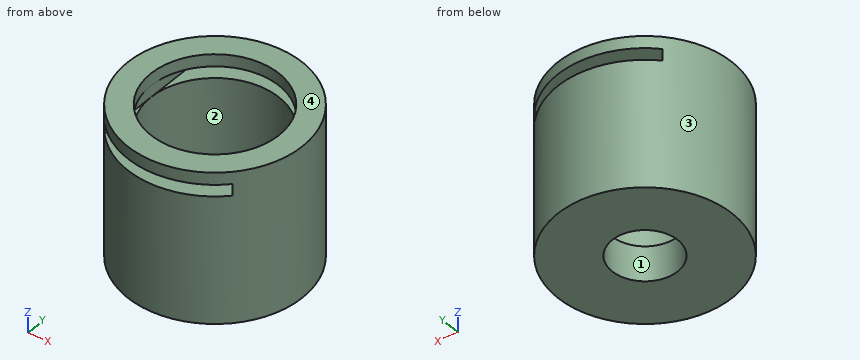
```python
from build123d import *

# Parameters (mm, degrees)
SKETCH1_R               = 15
BOSS_EXTRUDE5_DEPTH     = 26
SKETCH3_R               = 5.625
CUT_EXTRUDE2_DEPTH      = 34.555923471
SKETCH4_R               = 11
CUT_EXTRUDE3_DEPTH      = 20
CUT_EXTRUDE4_DEPTH      = 34.555923471
CUT_EXTRUDE4_DEPTH_BACK = 34.555923471
SKETCH6_W               = 22
SKETCH6_H               = 2
CUT_EXTRUDE6_START      = 6
SKETCH7_R               = 11
SKETCH7_R_2             = 9
CUT_EXTRUDE6_DEPTH      = 2


with BuildPart() as part:
    # Sketch1 → Boss-Extrude5 (new body)
    with BuildSketch(Plane.XY):
        Circle(SKETCH1_R)
    extrude(amount=BOSS_EXTRUDE5_DEPTH)

    # Sketch3 → Cut-Extrude2 (cut, through all)
    with BuildSketch(Plane.XY.offset(26)):
        Circle(SKETCH3_R)
    extrude(amount=-CUT_EXTRUDE2_DEPTH, mode=Mode.SUBTRACT)

    # Sketch4 → Cut-Extrude3 (cut)
    with BuildSketch(Plane.XY.offset(26)):
        Circle(SKETCH4_R)
    extrude(amount=-CUT_EXTRUDE3_DEPTH, mode=Mode.SUBTRACT)

    # Sketch6 → Cut-Extrude4 (cut, two sides: drawn at the far end of the back side and taken through both)
    with BuildSketch(Plane(origin=(0, 0, 0), x_dir=(1, 0, 0), z_dir=(0, 1, 0)).offset(-CUT_EXTRUDE4_DEPTH_BACK)):
        with Locations((0, -22.90958557)):
            Rectangle(SKETCH6_W, SKETCH6_H)
    extrude(amount=CUT_EXTRUDE4_DEPTH + CUT_EXTRUDE4_DEPTH_BACK, mode=Mode.SUBTRACT)

    # Sketch7 → Cut-Extrude6 (cut)
    with BuildSketch(Plane.XY.offset(CUT_EXTRUDE6_START)):
        Circle(SKETCH7_R)
        Circle(SKETCH7_R_2, mode=Mode.SUBTRACT)
    extrude(amount=-CUT_EXTRUDE6_DEPTH, mode=Mode.SUBTRACT)


solid = part.part
```
CAD build for the part. Positions are in the model's coordinates, mm. Face numbers are marked on the shaded views. Round coordinates to 2 decimals unless told otherwise and drop trailing zeros. Loops run counter-clockwise (first coordinate to the right, second up) from the corner with the lowest first, then second, coordinate; pieces in that order, holes last. Notation, with made-up numbers: M -17.5,-33 L 39.5,-33 A32 cw 39.5,4 Z; hole C 81.25,26 d9. An arc over 180 degrees is marked long. Use a Markdown table: item, result. Add a question column.
(1) Cut at C-C (z = 23.5). Give the cut face in (x, y), and give its area (3 significant figures).
(2) Cut at D-D (x = 9.5). Give the cut face in (y, z), and give its area (3 significant figures).
(3) Pull direction X, two halves, no side cores. Call the marked faces 1, 2, 3 and 4: +X half, -X half, draft (parallel to the pull), parting line (faces both ways), or undercut.
(4) Drill centre lines: line 1 (Y direction, x = 0, z = 4.6) (3 decimals); line 2 (Y direction, x = 0, z = 17.5); line 3 (Z direction, x = -6.25, y = -13.5). Where is each one in solid material? Low to high.
(5) Flat gauge pins, fed straight in: pin 1 (12 mm diameter, centred on x = 10, z = 10.5, fed in from +Y); pin 2 (12 mm diameter, centred on x = -2, y = -10, fed in from +Z); pin 3 (2 mm diameter, centred on y = 4.5, z = 23, fed in from +X); pin 4 (2 mm diameter, centred on y = 2, z = 15, fed in from +X). Where does each tip first touch, or does it go through?
(6) Cut at A-A (x = 0). Give the cut face in (y, z) (3 decimals).
Geometry says:
| question | item | result |
|---|---|---|
| 1 | outline | M -11,-10.2 L -11,10.2 A15 ccw Z; M 11,-10.2 A15 ccw 11,10.2 Z |
| 1 | area | 112 mm² |
| 2 | outline | M -11.61,0 L 11.61,0 L 11.61,21.91 L 5.55,21.91 L 5.55,4 L -5.55,4 L -5.55,21.91 L -11.61,21.91 Z; M -11.61,23.91 L -5.55,23.91 L -5.55,26 L -11.61,26 Z; M 5.55,23.91 L 11.61,23.91 L 11.61,26 L 5.55,26 Z |
| 2 | area | 335 mm² |
| 3 | face 1 | undercut |
| 3 | face 2 | undercut |
| 3 | face 3 | parting line |
| 3 | face 4 | draft |
| 4 | line 1 | y = -15 to -11, -9 to -5.625, 5.625 to 9, 11 to 15 |
| 4 | line 2 | y = -15 to -11, 11 to 15 |
| 4 | line 3 | z = 0 to 21.91, 23.91 to 26 |
| 5 | pin 1 | stops at y = 14.46 |
| 5 | pin 2 | stops at z = 26 |
| 5 | pin 3 | stops at x = 14.59 |
| 5 | pin 4 | stops at x = 14.97 |
| 6 | outline | M -15,0 L -5.625,0 L -5.625,6 L -9,6 L -9,4 L -11,4 L -11,21.91 L -15,21.91 Z; M -15,23.91 L -11,23.91 L -11,26 L -15,26 Z; M 5.625,0 L 15,0 L 15,21.91 L 11,21.91 L 11,4 L 9,4 L 9,6 L 5.625,6 Z; M 11,23.91 L 15,23.91 L 15,26 L 11,26 Z |
